```python
from build123d import *

# Parameters (mm, degrees)
F0_W     = 50.8
F0_H     = 50.8
F1_DEPTH = 635
F2_W     = 25.4
F2_H     = 19.05
F3_DEPTH = 25.4


with BuildPart() as f1:
    # F0 (on Top) → F1 (new body)
    with BuildSketch(Plane.XY):
        with Locations((25.4, 25.4)):
            Rectangle(F0_W, F0_H)
    extrude(amount=F1_DEPTH)

    # F2 (on face) → F3 (cut)
    with BuildSketch(Plane.XZ):
        with Locations((38.1, 60.325)):
            Rectangle(F2_W, F2_H)
        with Locations((38.1, 473.075)):
            Rectangle(F2_W, F2_H)
    extrude(amount=-F3_DEPTH, mode=Mode.SUBTRACT)


solid = f1.part
```
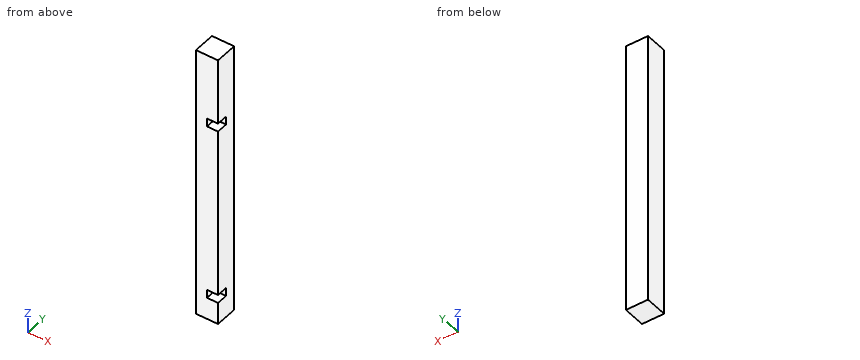
Verification items for the finished model (mm, model axes). Give positions to 0.01 mm unless a question says otherwise; leave off trailing zeros. Loops run counter-clockwise (first coordinate to the right, second up) from the corner with the lowest first, then second, coordinate; pieces in that order, holes last. Notation, with made-up numbers: M 57,69.5 L 70,69.5 A27 ccw 70,90.5 Z; hole C 31.25,70 d9. An arc over 180 degrees is marked long. Return JSON: item names as keys, results as strings.
1) Gauge pin test, flat ends, axial feed: P1, Ø7.5, axis at x = 33.5, y = 8.5, coming from the -Z side; P2, Ø9.5, axis at x = 43.5, z = 58, coming from the -Y side; P3, Ø5.5, axis at y = 7, z = 64, coming from the +X side. Record the tip position at first contact, or that the pin passes through.
Findings:
{"P1": "stops at z = 0", "P2": "stops at y = 25.4", "P3": "stops at x = 25.4"}
2) Section check A-A, the plane x = 43.5. Enter the section's corners in (y, z), and give its area (3 significant figures).
Findings:
{"outline": "M 0,0 L 50.8,0 L 50.8,635 L 0,635 L 0,482.6 L 25.4,482.6 L 25.4,463.55 L 0,463.55 L 0,69.85 L 25.4,69.85 L 25.4,50.8 L 0,50.8 Z", "area": "31,300 mm2"}
3) Section check B-B, the plane y = 12. Enter the section's corners in (x, z), and give its area (3 significant figures).
Findings:
{"outline": "M 0,0 L 50.8,0 L 50.8,50.8 L 25.4,50.8 L 25.4,69.85 L 50.8,69.85 L 50.8,463.55 L 25.4,463.55 L 25.4,482.6 L 50.8,482.6 L 50.8,635 L 0,635 Z", "area": "31,300 mm2"}
4) Material ranges on L1, parallel to Z at x = 45, y = 13.5; L2, parallel to Y at x = 42.5, z = 66, recorded low to high. Write a range as [from, to].
Findings:
{"L1": "z = [0, 50.8], [69.85, 463.55], [482.6, 635]", "L2": "y = [25.4, 50.8]"}
